Read the model definition and answer for the solid it produces. Units are mm, in the model's axes. A direction names the side the tool comes from. Give positions to 0.01 mm unless a question says otherwise; leave off trailing zeros. Order: outer loops, then holes, each group sorted by start corner. A loop starts at its lowest first (then second) coordinate and runs counter-clockwise, first axis right, second up.
Item 1: A cutting plane is placed at D-D (z = 4). Write down the section's boundary in (x, y).
Item 2: Find the intervals of material crossed by line 1 along Z through (x, y) = (8.25, 3.5); line 2 along X through (y, z) = (0.25, 2); line 3 along Z through (x, y) = (-7.5, -5.5), in increasing order.
Item 3: A cutting plane is placed at A-A (x = 0). Write down the section's boundary in (y, z), plus the area to 3 significant figures.
Item 4: Which of the six approach directions +Z, -Z, +X, -X, +Y, -Y give full straight-line access (tool end or side, diameter ignored) to faces 1 (the face through (4, -4, 3)), 2 (the face through (0, 0, 7.5))?
Item 5: A cutting plane is placed at C-C (z = 6.5). Write down the section's boundary in (x, y), plus the area to 3 significant figures.
Item 6: Given pin 1 Ø1.5 at (x, z) = (-7, 5.5) entering from +Y; pin 2 Ø1.5 at (y, z) = (7.5, 2) entering from +X; pin 3 Ø6 at (x, y) = (0, -7.5) entering from +Z, each flat-ended and moving along its own axis, determine where each tip first touches the part or whether it passes through.
from build123d import *

# Parameters (mm, degrees)
F0_R     = 9.5
F1_DEPTH = 3
F2_R     = 4
F3_DEPTH = 4.5
F4_SIZE  = 0.5
F5_R     = 4.55
F6_DEPTH = 1.5


with BuildPart() as f1:
    # F0 (on Top) → F1 (new body)
    with BuildSketch(Plane.XY):
        Circle(F0_R)
    extrude(amount=F1_DEPTH)

    # F2 (on face) → F3 (join)
    with BuildSketch(Plane.XY.offset(3)):
        Circle(F2_R)
    extrude(amount=F3_DEPTH)

    # F4
    f4_edges = [f1.edges().sort_by_distance(p)[0] for p in [
        (-4, 0, 7.5),
        (-9.5, 0, 3),
        (-9.5, 0, 0),
    ]]
    chamfer(f4_edges, length=F4_SIZE)

    # F5 (on face) → F6 (join)
    with BuildSketch(Plane.XY.offset(3)):
        Circle(F5_R)
    extrude(amount=F6_DEPTH)


solid = f1.part
Response values:
1. outline: circle Ø9.1 at (0, 0)
2. line 1: z = 0 to 3
2. line 2: x = -9.5 to 9.5
2. line 3: z = 0.3 to 2.7
3. outline: (-9.5, 0.5) - (-9, 0) - (9, 0) - (9.5, 0.5) - (9.5, 2.5) - (9, 3) - (4.55, 3) - (4.55, 4.5) - (4, 4.5) - (4, 7) - (3.5, 7.5) - (-3.5, 7.5) - (-4, 7) - (-4, 4.5) - (-4.55, 4.5) - (-4.55, 3) - (-9, 3) - (-9.5, 2.5) - close
3. area: 93.9 mm2
4. face 1: +Z
4. face 2: +Z, +X, -X, +Y, -Y
5. outline: circle Ø8 at (0, 0)
5. area: 50.3 mm2
6. pin 1: passes through
6. pin 2: stops at x = 6.68
6. pin 3: stops at z = 4.5
